```python
from build123d import *

# Parameters (mm, degrees)
SKETCH_1_W               = 42
SKETCH_1_H               = 42
EXTRUDE_1_DEPTH          = 60
CHAMFER_3_SIZE           = 3
SKETCH_2_R               = 11
EXTRUDE_2_DEPTH          = 1.8
SKETCH_3_R               = 2.5
EXTRUDE_3_DEPTH          = 24
SKETCH_4_OUTSIDE_W       = 64.576
SKETCH_4_OUTSIDE_H       = 64.576
CUT_EXTRUDE_1_DEPTH      = 36
FILLET_2_R               = 1
FILLET_3_R               = 0.2
CUT_EXTRUDE_START        = -15
CUT_EXTRUDE_5_DEPTH      = 15
CHAMFER_5_SIZE           = 0.3
CHAMFER_4_SIZE           = 0.5
SKETCH_6_R               = 1.3105
CUT_EXTRUDE_2_DEPTH      = 4.5
CUT_EXTRUDE_START_2      = -2
SKETCH_7_R               = 7.5
SKETCH_7_R_2             = 2.5
CUT_EXTRUDE_3_DEPTH      = 2
SKETCH_8_R               = 4.125
EXTRUDE_5_DEPTH          = 1.2
SKETCH_9_R               = 2.25
SKETCH_9_R_2             = 2.05
EXTRUDE_6_DEPTH          = 15.4
SKETCH_10_R              = 0.65
EXTRUDE_8_DEPTH          = 15.4
CUT_EXTRUDE_START_3      = -0.1
SKETCH_15_R              = 17.5
SKETCH_15_R_2            = 11
CUT_EXTRUDE_6_DEPTH      = 0.1
FILLET_4_R               = 0.3
PATTERN_CIRCULAR_3_COUNT = 4
SKETCH_20_W              = 88.292571494
SKETCH_20_H              = 79.893843274
CUT_EXTRUDE_13_DEPTH     = 15


with BuildPart() as part:
    # 草图1 → 凸台-拉伸1 (new body)
    with BuildSketch(Plane(origin=(0, 0, 0), x_dir=(1, 0, 0), z_dir=(0, 1, 0))):
        Rectangle(SKETCH_1_W, SKETCH_1_H)
    extrude(amount=EXTRUDE_1_DEPTH)

    # 倒角3
    chamfer_3_edges = [part.edges().sort_by_distance(p)[0] for p in [
        (-21, 30, -21),
        (21, 30, -21),
        (21, 30, 21),
        (-21, 30, 21),
    ]]
    chamfer(chamfer_3_edges, length=CHAMFER_3_SIZE)

    # 草图2 → 凸台-拉伸2 (add)
    with BuildSketch(Plane(origin=(0, 60, 0), x_dir=(1, 0, 0), z_dir=(0, 1, 0))):
        with Locations(Location((0, 0, 0), (0, 0, 270))):
            Circle(SKETCH_2_R)
    extrude(amount=EXTRUDE_2_DEPTH)

    # 草图3 → 凸台-拉伸3 (add)
    with BuildSketch(Plane(origin=(0, 60, 0), x_dir=(1, 0, 0), z_dir=(0, 1, 0))):
        with Locations(Location((0, 0, 0), (0, 0, 270))):
            Circle(SKETCH_3_R)
    extrude(amount=EXTRUDE_3_DEPTH)

    # 草图4 outside → 切除-拉伸1 (cut)
    with BuildSketch(Plane.XZ.offset(-12)):
        Rectangle(SKETCH_4_OUTSIDE_W, SKETCH_4_OUTSIDE_H)
        Polygon((15.471572875, 20.7), (-15.471572875, 20.7), (-20.7, 15.471572875), (-20.7, -15.471572875), (-15.471572875, -20.7), (15.471572875, -20.7), (20.7, -15.471572875), (20.7, 15.471572875), align=None, mode=Mode.SUBTRACT)
    extrude(amount=-CUT_EXTRUDE_1_DEPTH, mode=Mode.SUBTRACT)

    # 圆角2
    fillet_2_edges = [part.edges().sort_by_distance(p)[0] for p in [
        (-18, 6, -21),
        (18, 54, -21),
        (21, 54, 18),
        (21, 6, -18),
        (-18, 54, 21),
        (18, 6, 21),
        (-21, 54, -18),
        (-21, 6, 18),
        (-18, 54, -21),
        (-21, 6, -18),
        (-21, 54, 18),
        (-18, 6, 21),
        (18, 54, 21),
        (21, 6, 18),
        (21, 54, -18),
        (18, 6, -21),
    ]]
    fillet(fillet_2_edges, radius=FILLET_2_R)

    # 圆角3
    fillet_3_edges = [part.edges().sort_by_distance(p)[0] for p in [
        (21, 12, 0),
        (21, 0, 0),
        (0, 0, -21),
        (19.5, 0, -19.5),
        (19.5, 0, 19.5),
        (0, 0, 21),
        (-19.5, 0, 19.5),
        (-21, 0, 0),
        (-19.5, 0, -19.5),
        (-20.923879533, 0, -17.96846987),
        (-17.96846987, 0, -20.923879533),
        (17.96846987, 0, -20.923879533),
        (20.923879533, 0, -17.96846987),
        (-20.923879533, 0, 17.96846987),
        (-17.96846987, 0, 20.923879533),
        (17.96846987, 0, 20.923879533),
        (20.923879533, 0, 17.96846987),
        (19.5, 12, 19.5),
        (19.5, 12, -19.5),
        (0, 12, -21),
        (-19.5, 12, -19.5),
        (-21, 12, 0),
        (-19.5, 12, 19.5),
        (0, 12, 21),
        (-20.923879533, 12, -17.96846987),
        (-17.96846987, 12, -20.923879533),
        (17.96846987, 12, -20.923879533),
        (20.923879533, 12, -17.96846987),
        (-20.923879533, 12, 17.96846987),
        (-17.96846987, 12, 20.923879533),
        (17.96846987, 12, 20.923879533),
        (20.923879533, 12, 17.96846987),
        (0, 48, -21),
        (0, 60, -21),
        (21, 60, 0),
        (19.5, 60, -19.5),
        (-19.5, 60, -19.5),
        (-21, 60, 0),
        (-19.5, 60, 19.5),
        (0, 60, 21),
        (19.5, 60, 19.5),
        (-20.923879533, 60, 17.96846987),
        (-17.96846987, 60, 20.923879533),
        (17.96846987, 60, 20.923879533),
        (20.923879533, 60, 17.96846987),
        (17.96846987, 60, -20.923879533),
        (20.923879533, 60, -17.96846987),
        (-20.923879533, 60, -17.96846987),
        (-17.96846987, 60, -20.923879533),
        (-19.5, 48, -19.5),
        (0, 48, 21),
        (-19.5, 48, 19.5),
        (-21, 48, 0),
        (19.5, 48, -19.5),
        (21, 48, 0),
        (19.5, 48, 19.5),
        (-20.923879533, 48, 17.96846987),
        (-17.96846987, 48, 20.923879533),
        (17.96846987, 48, 20.923879533),
        (20.923879533, 48, 17.96846987),
        (17.96846987, 48, -20.923879533),
        (20.923879533, 48, -17.96846987),
        (-20.923879533, 48, -17.96846987),
        (-17.96846987, 48, -20.923879533),
    ]]
    fillet(fillet_3_edges, radius=FILLET_3_R)

    # 草图14 → 切除-拉伸5 (cut)
    with BuildSketch(Plane(origin=(0, 84, 0), x_dir=(1, 0, 0), z_dir=(0, 1, 0)).offset(CUT_EXTRUDE_START)):
        with BuildLine():
            Line((-2, 1.5), (-2, -1.5))
            ThreePointArc((-2, -1.5), (-2.5, 0), (-2, 1.5))
        make_face()
    extrude(amount=CUT_EXTRUDE_5_DEPTH, mode=Mode.SUBTRACT)

    # 倒角5
    chamfer_5_edges = [part.edges().sort_by_distance(p)[0] for p in [
        (2.236067977, 84, -1.118033989),
    ]]
    chamfer(chamfer_5_edges, length=CHAMFER_5_SIZE)

    # 倒角4
    chamfer_4_edges = [part.edges().sort_by_distance(p)[0] for p in [
        (-2, 69, 0),
    ]]
    chamfer(chamfer_4_edges, length=CHAMFER_4_SIZE - 0.0001)  # a hair under: the kernel refuses the full size

    # 草图6 → 切除-拉伸2 (cut)
    with BuildSketch(Plane(origin=(0, 60, 0), x_dir=(1, 0, 0), z_dir=(0, 1, 0))):
        with Locations(Location((-15.5, 15.5, 0), (0, 0, 270))):
            Circle(SKETCH_6_R)
        with Locations(Location((15.5, 15.5, 0), (0, 0, 90))):
            Circle(SKETCH_6_R)
        with Locations(Location((15.5, -15.5, 0), (0, 0, 270))):
            Circle(SKETCH_6_R)
        with Locations(Location((-15.5, -15.5, 0), (0, 0, 90))):
            Circle(SKETCH_6_R)
    extrude(amount=-CUT_EXTRUDE_2_DEPTH, mode=Mode.SUBTRACT)

    # 草图7 → 切除-拉伸3 (cut)
    with BuildSketch(Plane(origin=(0, 61.8, 0), x_dir=(1, 0, 0), z_dir=(0, 1, 0)).offset(CUT_EXTRUDE_START_2)):
        with Locations(Location((0, 0, 0), (0, 0, 270))):
            Circle(SKETCH_7_R)
        with Locations(Location((0, 0, 0), (0, 0, 143.130102354))):
            Circle(SKETCH_7_R_2, mode=Mode.SUBTRACT)
    extrude(amount=CUT_EXTRUDE_3_DEPTH, mode=Mode.SUBTRACT)

    # 草图8 → 凸台-拉伸5 (add)
    with BuildSketch(Plane(origin=(21, 0, 0), x_dir=(0, 0, -1), z_dir=(1, 0, 0))):
        with Locations(Location((0, 6, 0), (0, 0, 180))):
            Circle(SKETCH_8_R)
    extrude(amount=EXTRUDE_5_DEPTH)

    # 草图9 → 凸台-拉伸6 (add)
    with BuildSketch(Plane(origin=(22.2, 0, 0), x_dir=(0, 0, -1), z_dir=(1, 0, 0))):
        with Locations(Location((0, 6, 0), (0, 0, 180))):
            Circle(SKETCH_9_R)
        with Locations(Location((0, 6, 0), (0, 0, 180))):
            Circle(SKETCH_9_R_2, mode=Mode.SUBTRACT)
    extrude(amount=EXTRUDE_6_DEPTH)

    # 草图10 → 凸台-拉伸8 (add)
    with BuildSketch(Plane(origin=(22.2, 0, 0), x_dir=(0, 0, -1), z_dir=(1, 0, 0))):
        with Locations((0.952627944, 6.55)):
            Circle(SKETCH_10_R)
    extrude_8 = extrude(amount=EXTRUDE_8_DEPTH)

    # 草图15 → 切除-拉伸6 (cut)
    with BuildSketch(Plane(origin=(0, 60, 0), x_dir=(1, 0, 0), z_dir=(0, 1, 0)).offset(CUT_EXTRUDE_START_3)):
        with Locations(Location((0, 0, 0), (0, 0, 270))):
            Circle(SKETCH_15_R)
        with Locations(Location((0, 0, 0), (0, 0, 270))):
            Circle(SKETCH_15_R_2, mode=Mode.SUBTRACT)
    extrude(amount=CUT_EXTRUDE_6_DEPTH, mode=Mode.SUBTRACT)

    # 圆角4
    fillet_4_edges = [part.edges().sort_by_distance(p)[0] for p in [
        (0, 61.8, -11),
        (0, 61.8, -7.5),
    ]]
    fillet(fillet_4_edges, radius=FILLET_4_R)

    # 阵列(圆周)3: 凸台-拉伸8 ×4 about axis
    pattern_circular_3_axis = Axis((0, 6, 0), (1, 0, 0))
    for i in range(1, PATTERN_CIRCULAR_3_COUNT):
        add(extrude_8.rotate(pattern_circular_3_axis, i * 360 / PATTERN_CIRCULAR_3_COUNT))

    # 草图20 → 切除-拉伸13 (cut)
    with BuildSketch(Plane.XZ):
        Rectangle(SKETCH_20_W, SKETCH_20_H)
    extrude(amount=-CUT_EXTRUDE_13_DEPTH, mode=Mode.SUBTRACT)


solid = part.part
```
Design review of the part built by this model. Coordinates are the model's own, in mm. A direction names the side the tool comes from. Round coordinates to 2 decimals unless told otherwise and drop trailing zeros. Write each loop counter-clockwise with the first axis right and the second up, starting at its lowest first coordinate (ties: lowest second). Pieces come first, ordered by that corner, then holes. Notation, with made-up numbers: (39, -39) -> (71, -39) arc R13 cw to (71, -26) -> close; hole circle Ø6 at (-20.75, 69). An arc over 180 degrees is marked (long way). Write item = value, one per line. Start each with the question number.
1) Take a section at A-A, the plane y = 45.5. State the section outline as (x, z) points.
2) Mouldability with a two-part tool opening along X and no side actions: class faces 1 (the face through (-19.474, 59.943, 19.441)), 2 (the face through (19.441, 59.943, 19.474)), 3 (the face through (-16, 55.5, 16)) as +X half, -X half, draft (parallel to the pull), parting line (faces both ways), or undercut.
3) Tool access review of faces 4 (the face through (0, 31, 20.7)), 5 (the face through (-8, 59.9, -8)), 6 (the face through (0, 84, 0)): name each direction out of +Z, -Z, +X, -X, +Y, -Y from which nothing blocks a thin tool from reaching the whole face with its end or side.
4) Wall thickness on probe 1 along X at (y, z) = (56.55, 15.5); probe 2 along Y at (x, z) = (14.5, 16); probe 3 along X at (y, z) = (56, -15): over which ranges is each line inside the solid? List them lowest first. Write a range as from..to.
5) Take a section at C-C, the plane y = 64. State the section outline as (x, z) points, plus the area to 3 significant figures.
6) Take a section at B-B, the plane y = 77.5. State the section outline as (x, z) points, plus the area to 3 significant figures.
7) Clearance check with flat-ended pins moving along their axes: pin 1 (3 mm diameter, centred on x = -15.5, z = -15.5, fed in from +Y); pin 2 (0.8 mm diameter, centred on x = 15.5, z = 15.5, fed in from +Y); pin 3 (9.5 mm diameter, centred on x = -2.5, y = 33, fed in from -Z); pin 4 (4 mm diameter, centred on y = 47, z = 1, fed in from -X). State where each tip first meets the part, or that it passes through.
Results list:
q1.outline = (-20.7, -15.47) -> (-15.47, -20.7) -> (15.47, -20.7) -> (20.7, -15.47) -> (20.7, 15.47) -> (15.47, 20.7) -> (-15.47, 20.7) -> (-20.7, 15.47) -> close
q2.face_1 = -X half
q2.face_2 = +X half
q2.face_3 = undercut
q3.face_4 = +Z, +X, -X, -Y
q3.face_5 = +Y
q3.face_6 = +Z, -Z, +X, -X, +Y
q4.probe_1 = -21..-16.81, -14.19..14.19, 16.81..21
q4.probe_2 = 15..55.5
q4.probe_3 = -21..-16.71, -14.29..14.29, 16.71..21
q5.outline = circle Ø5 at (0, 0)
q5.area = 19.6 mm²
q6.outline = (-2, -1.5) arc R2.5 ccw (long way) to (-2, 1.5) -> close
q6.area = 18.6 mm²
q7.pin_1 = 60
q7.pin_2 = 55.5
q7.pin_3 = -20.7
q7.pin_4 = -21
